Verification items for the finished model (mm, model axes). Round coordinates to 2 decimals unless told otherwise and drop trailing zeros. Loops run counter-clockwise (first coordinate to the right, second up) from the corner with the lowest first, then second, coordinate; pieces in that order, holes last. Notation, with made-up numbers: M 6,38.25 L 58,38.25 A24 ccw 58,55.25 Z; hole C 27.25,33.25 d4. An arc over 180 degrees is marked long. Answer as CSV lines item,"result".
```python
from build123d import *

# Parameters (mm, degrees)
BOSS_EXTRUDE1_DEPTH = 10
CUT_EXTRUDE1_REACH  = 179.059
SKETCH2_R           = 2.05
BOSS_EXTRUDE2_DEPTH = 10
BOSS_EXTRUDE3_DEPTH = 10
SKETCH5_R           = 3.5
CUT_EXTRUDE2_DEPTH  = 4
SKETCH6_R           = 3.75
CUT_EXTRUDE4_DEPTH  = 223.256608451


# Read off the part's stored shape, not the designer's step: moBlkMgr[DitRB1]
with BuildPart() as part:
    # Sketch1 → Boss-Extrude1 (new body)
    with BuildSketch(Plane(origin=(0, 0, 0), x_dir=(1, 0, 0), z_dir=(0, 1, 0))):
        Polygon((-96.715728753, 125), (-125, 96.715728753), (-125, -96.715728753), (-96.715728753, -125), (96.715728753, -125), (125, -96.715728753), (125, 96.715728753), (96.715728753, 125), align=None)
    extrude(amount=BOSS_EXTRUDE1_DEPTH)

    # Sketch2 → Cut-Extrude1 (cut, up to next)
    with BuildSketch(Plane(origin=(0, 10, 0), x_dir=(1, 0, 0), z_dir=(0, 1, 0)), mode=Mode.PRIVATE) as cut_extrude1_sk1:
        with Locations(Location((-97.069282143, -75.856078708, 0), (0, 0, 270))):
            Circle(SKETCH2_R)
    cut_extrude1_tool1 = extrude(cut_extrude1_sk1.sketch, amount=-CUT_EXTRUDE1_REACH, mode=Mode.PRIVATE) & part.part
    # Sketch2 → Cut-Extrude1 (cut, up to next)
    with BuildSketch(Plane(origin=(0, 10, 0), x_dir=(1, 0, 0), z_dir=(0, 1, 0)), mode=Mode.PRIVATE) as cut_extrude1_sk2:
        with Locations(Location((-114.039844892, -92.826641456, 0), (0, 0, 270))):
            Circle(SKETCH2_R)
    cut_extrude1_tool2 = extrude(cut_extrude1_sk2.sketch, amount=-CUT_EXTRUDE1_REACH, mode=Mode.PRIVATE) & part.part
    # Sketch2 → Cut-Extrude1 (cut, up to next)
    with BuildSketch(Plane(origin=(0, 10, 0), x_dir=(1, 0, 0), z_dir=(0, 1, 0)), mode=Mode.PRIVATE) as cut_extrude1_sk3:
        with Locations(Location((-75.856078708, -97.069282143, 0), (0, 0, 90))):
            Circle(SKETCH2_R)
    cut_extrude1_tool3 = extrude(cut_extrude1_sk3.sketch, amount=-CUT_EXTRUDE1_REACH, mode=Mode.PRIVATE) & part.part
    # Sketch2 → Cut-Extrude1 (cut, up to next)
    with BuildSketch(Plane(origin=(0, 10, 0), x_dir=(1, 0, 0), z_dir=(0, 1, 0)), mode=Mode.PRIVATE) as cut_extrude1_sk4:
        with Locations(Location((-92.826641456, -114.039844892, 0), (0, 0, 90))):
            Circle(SKETCH2_R)
    cut_extrude1_tool4 = extrude(cut_extrude1_sk4.sketch, amount=-CUT_EXTRUDE1_REACH, mode=Mode.PRIVATE) & part.part
    # Sketch2 → Cut-Extrude1 (cut, up to next)
    with BuildSketch(Plane(origin=(0, 10, 0), x_dir=(1, 0, 0), z_dir=(0, 1, 0)), mode=Mode.PRIVATE) as cut_extrude1_sk5:
        with Locations(Location((-75.856078708, 97.069282143, 0), (0, 0, 270))):
            Circle(SKETCH2_R)
    cut_extrude1_tool5 = extrude(cut_extrude1_sk5.sketch, amount=-CUT_EXTRUDE1_REACH, mode=Mode.PRIVATE) & part.part
    # Sketch2 → Cut-Extrude1 (cut, up to next)
    with BuildSketch(Plane(origin=(0, 10, 0), x_dir=(1, 0, 0), z_dir=(0, 1, 0)), mode=Mode.PRIVATE) as cut_extrude1_sk6:
        with Locations(Location((-92.826641456, 114.039844892, 0), (0, 0, 270))):
            Circle(SKETCH2_R)
    cut_extrude1_tool6 = extrude(cut_extrude1_sk6.sketch, amount=-CUT_EXTRUDE1_REACH, mode=Mode.PRIVATE) & part.part
    # Sketch2 → Cut-Extrude1 (cut, up to next)
    with BuildSketch(Plane(origin=(0, 10, 0), x_dir=(1, 0, 0), z_dir=(0, 1, 0)), mode=Mode.PRIVATE) as cut_extrude1_sk7:
        with Locations(Location((-114.039844892, 92.826641456, 0), (0, 0, 90))):
            Circle(SKETCH2_R)
    cut_extrude1_tool7 = extrude(cut_extrude1_sk7.sketch, amount=-CUT_EXTRUDE1_REACH, mode=Mode.PRIVATE) & part.part
    # Sketch2 → Cut-Extrude1 (cut, up to next)
    with BuildSketch(Plane(origin=(0, 10, 0), x_dir=(1, 0, 0), z_dir=(0, 1, 0)), mode=Mode.PRIVATE) as cut_extrude1_sk8:
        with Locations(Location((-97.069282143, 75.856078708, 0), (0, 0, 90))):
            Circle(SKETCH2_R)
    cut_extrude1_tool8 = extrude(cut_extrude1_sk8.sketch, amount=-CUT_EXTRUDE1_REACH, mode=Mode.PRIVATE) & part.part
    # Sketch2 → Cut-Extrude1 (cut, up to next)
    with BuildSketch(Plane(origin=(0, 10, 0), x_dir=(1, 0, 0), z_dir=(0, 1, 0)), mode=Mode.PRIVATE) as cut_extrude1_sk9:
        with Locations(Location((97.069282143, 75.856078708, 0), (0, 0, 270))):
            Circle(SKETCH2_R)
    cut_extrude1_tool9 = extrude(cut_extrude1_sk9.sketch, amount=-CUT_EXTRUDE1_REACH, mode=Mode.PRIVATE) & part.part
    # Sketch2 → Cut-Extrude1 (cut, up to next)
    with BuildSketch(Plane(origin=(0, 10, 0), x_dir=(1, 0, 0), z_dir=(0, 1, 0)), mode=Mode.PRIVATE) as cut_extrude1_sk10:
        with Locations(Location((114.039844892, 92.826641456, 0), (0, 0, 270))):
            Circle(SKETCH2_R)
    cut_extrude1_tool10 = extrude(cut_extrude1_sk10.sketch, amount=-CUT_EXTRUDE1_REACH, mode=Mode.PRIVATE) & part.part
    # Sketch2 → Cut-Extrude1 (cut, up to next)
    with BuildSketch(Plane(origin=(0, 10, 0), x_dir=(1, 0, 0), z_dir=(0, 1, 0)), mode=Mode.PRIVATE) as cut_extrude1_sk11:
        with Locations(Location((92.826641456, 114.039844892, 0), (0, 0, 90))):
            Circle(SKETCH2_R)
    cut_extrude1_tool11 = extrude(cut_extrude1_sk11.sketch, amount=-CUT_EXTRUDE1_REACH, mode=Mode.PRIVATE) & part.part
    # Sketch2 → Cut-Extrude1 (cut, up to next)
    with BuildSketch(Plane(origin=(0, 10, 0), x_dir=(1, 0, 0), z_dir=(0, 1, 0)), mode=Mode.PRIVATE) as cut_extrude1_sk12:
        with Locations(Location((75.856078708, 97.069282143, 0), (0, 0, 90))):
            Circle(SKETCH2_R)
    cut_extrude1_tool12 = extrude(cut_extrude1_sk12.sketch, amount=-CUT_EXTRUDE1_REACH, mode=Mode.PRIVATE) & part.part
    # Sketch2 → Cut-Extrude1 (cut, up to next)
    with BuildSketch(Plane(origin=(0, 10, 0), x_dir=(1, 0, 0), z_dir=(0, 1, 0)), mode=Mode.PRIVATE) as cut_extrude1_sk13:
        with Locations(Location((75.856078708, -97.069282143, 0), (0, 0, 270))):
            Circle(SKETCH2_R)
    cut_extrude1_tool13 = extrude(cut_extrude1_sk13.sketch, amount=-CUT_EXTRUDE1_REACH, mode=Mode.PRIVATE) & part.part
    # Sketch2 → Cut-Extrude1 (cut, up to next)
    with BuildSketch(Plane(origin=(0, 10, 0), x_dir=(1, 0, 0), z_dir=(0, 1, 0)), mode=Mode.PRIVATE) as cut_extrude1_sk14:
        with Locations(Location((92.826641456, -114.039844892, 0), (0, 0, 270))):
            Circle(SKETCH2_R)
    cut_extrude1_tool14 = extrude(cut_extrude1_sk14.sketch, amount=-CUT_EXTRUDE1_REACH, mode=Mode.PRIVATE) & part.part
    # Sketch2 → Cut-Extrude1 (cut, up to next)
    with BuildSketch(Plane(origin=(0, 10, 0), x_dir=(1, 0, 0), z_dir=(0, 1, 0)), mode=Mode.PRIVATE) as cut_extrude1_sk15:
        with Locations(Location((114.039844892, -92.826641456, 0), (0, 0, 90))):
            Circle(SKETCH2_R)
    cut_extrude1_tool15 = extrude(cut_extrude1_sk15.sketch, amount=-CUT_EXTRUDE1_REACH, mode=Mode.PRIVATE) & part.part
    # Sketch2 → Cut-Extrude1 (cut, up to next)
    with BuildSketch(Plane(origin=(0, 10, 0), x_dir=(1, 0, 0), z_dir=(0, 1, 0)), mode=Mode.PRIVATE) as cut_extrude1_sk16:
        with Locations(Location((97.069282143, -75.856078708, 0), (0, 0, 90))):
            Circle(SKETCH2_R)
    cut_extrude1_tool16 = extrude(cut_extrude1_sk16.sketch, amount=-CUT_EXTRUDE1_REACH, mode=Mode.PRIVATE) & part.part
    add(cut_extrude1_tool1.solids().sort_by_distance((-97.069282, 10, 75.856079))[0], mode=Mode.SUBTRACT)
    add(cut_extrude1_tool2.solids().sort_by_distance((-114.039845, 10, 92.826641))[0], mode=Mode.SUBTRACT)
    add(cut_extrude1_tool3.solids().sort_by_distance((-75.856079, 10, 97.069282))[0], mode=Mode.SUBTRACT)
    add(cut_extrude1_tool4.solids().sort_by_distance((-92.826641, 10, 114.039845))[0], mode=Mode.SUBTRACT)
    add(cut_extrude1_tool5.solids().sort_by_distance((-75.856079, 10, -97.069282))[0], mode=Mode.SUBTRACT)
    add(cut_extrude1_tool6.solids().sort_by_distance((-92.826641, 10, -114.039845))[0], mode=Mode.SUBTRACT)
    add(cut_extrude1_tool7.solids().sort_by_distance((-114.039845, 10, -92.826641))[0], mode=Mode.SUBTRACT)
    add(cut_extrude1_tool8.solids().sort_by_distance((-97.069282, 10, -75.856079))[0], mode=Mode.SUBTRACT)
    add(cut_extrude1_tool9.solids().sort_by_distance((97.069282, 10, -75.856079))[0], mode=Mode.SUBTRACT)
    add(cut_extrude1_tool10.solids().sort_by_distance((114.039845, 10, -92.826641))[0], mode=Mode.SUBTRACT)
    add(cut_extrude1_tool11.solids().sort_by_distance((92.826641, 10, -114.039845))[0], mode=Mode.SUBTRACT)
    add(cut_extrude1_tool12.solids().sort_by_distance((75.856079, 10, -97.069282))[0], mode=Mode.SUBTRACT)
    add(cut_extrude1_tool13.solids().sort_by_distance((75.856079, 10, 97.069282))[0], mode=Mode.SUBTRACT)
    add(cut_extrude1_tool14.solids().sort_by_distance((92.826641, 10, 114.039845))[0], mode=Mode.SUBTRACT)
    add(cut_extrude1_tool15.solids().sort_by_distance((114.039845, 10, 92.826641))[0], mode=Mode.SUBTRACT)
    add(cut_extrude1_tool16.solids().sort_by_distance((97.069282, 10, 75.856079))[0], mode=Mode.SUBTRACT)

    # Sketch3 → Boss-Extrude2 (add)
    with BuildSketch(Plane(origin=(0, 10, 0), x_dir=(1, 0, 0), z_dir=(0, 1, 0))):
        Polygon((-125, 96.715728753), (-157, 64.715728753), (-157, -64.715728753), (-125, -96.715728753), align=None)
        Polygon((64.715728753, 157), (-64.715728753, 157), (-96.715728753, 125), (96.715728753, 125), align=None)
        Polygon((157, -64.715728753), (157, 64.715728753), (125, 96.715728753), (125, -96.715728753), align=None)
        Polygon((-64.715728753, -157), (64.715728753, -157), (96.715728753, -125), (-96.715728753, -125), align=None)
    extrude(amount=-BOSS_EXTRUDE2_DEPTH)

    # Sketch4 → Boss-Extrude3 (add)
    with BuildSketch(Plane(origin=(0, 10, 0), x_dir=(1, 0, 0), z_dir=(0, 1, 0))):
        Polygon((-157, 64.715728753), (-64.715728753, 157), (-117.04163056, 157), (-157, 117.04163056), align=None)
        Polygon((64.715728753, 157), (157, 64.715728753), (157, 117.04163056), (117.04163056, 157), align=None)
        Polygon((157, -64.715728753), (64.715728753, -157), (117.04163056, -157), (157, -117.04163056), align=None)
        Polygon((-64.715728753, -157), (-157, -64.715728753), (-157, -117.04163056), (-117.04163056, -157), align=None)
    extrude(amount=-BOSS_EXTRUDE3_DEPTH)

    # Sketch5 → Cut-Extrude2 (cut)
    with BuildSketch(Plane.XZ):
        with Locations(Location((-114.039844892, 92.826641456, 0), (0, 0, 270))):
            Circle(SKETCH5_R)
        with Locations(Location((-92.826641456, 114.039844892, 0), (0, 0, 270))):
            Circle(SKETCH5_R)
        with Locations(Location((-75.856078708, 97.069282143, 0), (0, 0, 270))):
            Circle(SKETCH5_R)
        with Locations(Location((-97.069282143, 75.856078708, 0), (0, 0, 270))):
            Circle(SKETCH5_R)
        with Locations(Location((114.039844892, 92.826641456, 0), (0, 0, 270))):
            Circle(SKETCH5_R)
        with Locations(Location((92.826641456, 114.039844892, 0), (0, 0, 270))):
            Circle(SKETCH5_R)
        with Locations(Location((75.856078708, 97.069282143, 0), (0, 0, 270))):
            Circle(SKETCH5_R)
        with Locations(Location((97.069282143, 75.856078708, 0), (0, 0, 270))):
            Circle(SKETCH5_R)
        with Locations(Location((92.826641456, -114.039844892, 0), (0, 0, 270))):
            Circle(SKETCH5_R)
        with Locations(Location((114.039844892, -92.826641456, 0), (0, 0, 270))):
            Circle(SKETCH5_R)
        with Locations(Location((97.069282143, -75.856078708, 0), (0, 0, 270))):
            Circle(SKETCH5_R)
        with Locations(Location((75.856078708, -97.069282143, 0), (0, 0, 270))):
            Circle(SKETCH5_R)
        with Locations(Location((-114.039844892, -92.826641456, 0), (0, 0, 270))):
            Circle(SKETCH5_R)
        with Locations(Location((-92.826641456, -114.039844892, 0), (0, 0, 270))):
            Circle(SKETCH5_R)
        with Locations(Location((-75.856078708, -97.069282143, 0), (0, 0, 270))):
            Circle(SKETCH5_R)
        with Locations(Location((-97.069282143, -75.856078708, 0), (0, 0, 270))):
            Circle(SKETCH5_R)
    extrude(amount=-CUT_EXTRUDE2_DEPTH, mode=Mode.SUBTRACT)

    # Sketch6 → Cut-Extrude4 (cut, through all)
    with BuildSketch(Plane.XZ):
        with Locations(Location((-59.5, -17.1, 0), (0, 0, 270))):
            Circle(SKETCH6_R)
        with Locations(Location((-14.5, -17.1, 0), (0, 0, 270))):
            Circle(SKETCH6_R)
        with Locations(Location((-14.5, -62.1, 0), (0, 0, 270))):
            Circle(SKETCH6_R)
        with Locations(Location((-59.5, -62.1, 0), (0, 0, 270))):
            Circle(SKETCH6_R)
    extrude(amount=-CUT_EXTRUDE4_DEPTH, mode=Mode.SUBTRACT)


solid = part.part
```
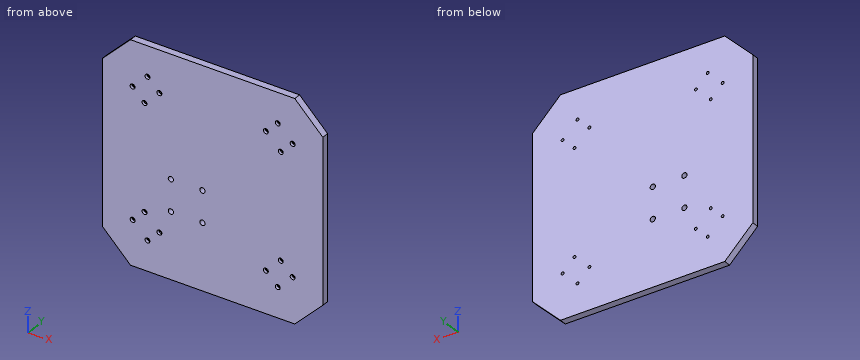
1) Material ranges on probe 1 along Z at (x, y) = (-60, 4.75); probe 2 along X at (y, z) = (7.75, -95.5); probe 3 along X at (y, z) = (3.5, -62.1), recorded low to high.
Here are the results:
probe 1,"z = -157 to -65.82, -58.38 to -20.82, -13.38 to 157"
probe 2,"x = -157 to -77.18, -74.54 to 74.54, 77.18 to 157"
probe 3,"x = -157 to -63.25, -55.75 to -18.25, -10.75 to 157"
2) Go/stop test with flat-tipped pins: pin 1 (3.5 mm diameter, centred on x = 92, z = -114, fed in from -Y); pin 2 (3.5 mm diameter, centred on x = -97.07, z = 75.86, fed in from -Y). Record where each tip stops, or that it passes through.
Here are the results:
pin 1,"stops at y = 4"
pin 2,"passes through"
3) Section check B-B (x = -59.5). Record the cut outline in (y, z).
Here are the results:
outline,"M 0,-157 L 10,-157 L 10,-65.85 L 0,-65.85 Z; M 0,-58.35 L 10,-58.35 L 10,-20.85 L 0,-20.85 Z; M 0,-13.35 L 10,-13.35 L 10,157 L 0,157 Z"
4) Section check A-A (z = -17.1). Record the cut outline in (x, y).
Here are the results:
outline,"M -157,0 L -63.25,0 L -63.25,10 L -157,10 Z; M -55.75,0 L -18.25,0 L -18.25,10 L -55.75,10 Z; M -10.75,0 L 157,0 L 157,10 L -10.75,10 Z"
5) Section check C-C (y = 2). State how many separate pieces and enclosed holes the cut face has, plus the area to 3 significant figures.
Here are the results:
separate pieces,"1"
enclosed holes,"20"
area,"94,600 mm^2"
